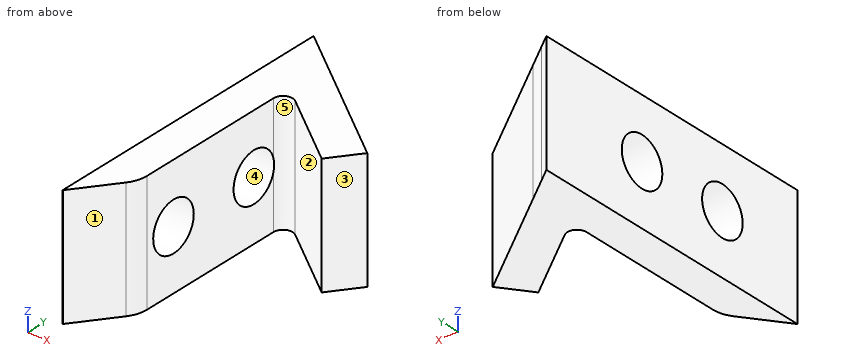
from build123d import *

# Parameters (mm, degrees)
BOSS_EXTRUDE1_DEPTH = 10
FILLET1_R           = 0.8
FILLET2_R           = 2.5
SKETCH6_R           = 2.02
CUT_EXTRUDE1_DEPTH  = 4


with BuildPart() as part:
    # Sketch2 → Boss-Extrude1 (new body)
    with BuildSketch(Plane.XY):
        Polygon((0, 21.259357975), (0, 0.022383201), (0.016670773, 0.022383201), (3, 4.02798368), (3, 19.024989439), align=None)
        Polygon((0, 22.637274757), (0, 21.259357975), (3, 19.024989439), (3, 22.765631464), (1.131871138, 24.156994247), align=None)
        Polygon((3, 22.765631464), (3, 19.024989439), (10.184363913, 13.674150545), (11.976330523, 16.080154633), align=None)
        Polygon((0, 25), (0, 22.637274757), (1.131871138, 24.156994247), align=None)
    extrude(amount=BOSS_EXTRUDE1_DEPTH)

    # Fillet1
    fillet1_edges = [part.edges().sort_by_distance(p)[0] for p in [
        (3, 19.024989439, 5),
    ]]
    fillet(fillet1_edges, radius=FILLET1_R)

    # Fillet2
    fillet2_edges = [part.edges().sort_by_distance(p)[0] for p in [
        (3, 4.02798368, 5),
    ]]
    fillet(fillet2_edges, radius=FILLET2_R)

    # Sketch6 → Cut-Extrude1 (cut)
    with BuildSketch(Plane.ZY):
        with Locations((5, 15.476622616)):
            Circle(SKETCH6_R)
        with Locations((5, 7.476622616)):
            Circle(SKETCH6_R)
    extrude(amount=-CUT_EXTRUDE1_DEPTH, mode=Mode.SUBTRACT)


solid = part.part
Design review of the part built by this model. Coordinates are the model's own, in mm. Face numbers are marked on the shaded views. A direction names the side the tool comes from. Round coordinates to 2 decimals unless told otherwise and drop trailing zeros. Write each loop counter-clockwise with the first axis right and the second up, starting at its lowest first coordinate (ties: lowest second). Pieces come first, ordered by that corner, then holes. Notation, with made-up numbers: (76, 77) -> (101, 77) arc R30 ccw to (101, 99) -> close; hole circle Ø9 at (43.25, -20). An arc over 180 degrees is marked (long way). One line per item, written item: value. Start each with the question number.
Q1. Insertion check: P1, Ø4.5, axis at y = 15.48, z = 5, coming from the +X side; P2, Ø2, axis at x = 3, z = 8.5, coming from the -Y side; P3, Ø6, axis at y = 4.5, z = 3.5, coming from the +X side. Each pin has a flat end and moves straight along its axis. Give the tip position at first contact, or say it passes through.
Q2. To check wall thickness, follow probe 1 along Y at (x, z) = (1.4, 5); probe 2 along Y at (x, z) = (2.25, 5); probe 3 along X at (y, z) = (9.5, 8). State the ranges of each line that lie inside material, in increasing order.
Q3. The part is to be moulded in two halves that separate along X. For the marked faces 3, 4 and 5, say which applies: pulls with the +X half, pulls with the -X half, needs draft (parallel to the pull), parting line crosses it, or undercut.
Q4. Add section B-B (y = 14.5). Give the boundary of the cut face in (x, z), then the cut area to 3 significant figures.
Q5. Add section D-D (z = 9.25). Give the boundary of the cut face in (x, y) (3 decimals).
Q6. Tool access review of the marked faces 1 and 2: name each direction out of +Z, -Z, +X, -X, +Y, -Y from which nothing blocks a thin tool from reaching the whole face with its end or side.
Q7. Add section C-C (y = 6). Give the boundary of the cut face in (x, z).
Q8. Add section A-A (z = 5). Give the boundary of the cut face in (x, y) (3 decimals), then the cut area to 3 significant figures.
Response:
1. P1: stops at x = 11.98
1. P2: stops at y = 2.69
1. P3: stops at x = 3
2. probe 1: y = 1.88 to 5.46, 9.5 to 13.46, 17.5 to 23.96
2. probe 2: y = 3.02 to 5.46, 9.5 to 13.46, 17.5 to 23.32
2. probe 3: x = 0 to 3
3. face 3: pulls with the +X half
3. face 4: needs draft
3. face 5: undercut
4. outline: (0, 0) -> (3, 0) -> (3, 3.23) -> (0, 3.23) -> close; (0, 6.77) -> (3, 6.77) -> (3, 10) -> (0, 10) -> close; (9.08, 0) -> (10.8, 0) -> (10.8, 10) -> (9.08, 10) -> close
4. area: 36.6 mm^2
5. outline: (0, 0.022) -> (0.017, 0.022) -> (2.505, 3.363) arc R2.5 ccw to (3, 4.857) -> (3, 17.432) arc R0.8 cw to (4.278, 18.073) -> (10.184, 13.674) -> (11.976, 16.08) -> (0, 25) -> close
6. face 1: +Z, -Z, +X, -Y
6. face 2: +Z, -Z, -Y
7. outline: (0, 0) -> (3, 0) -> (3, 3.62) -> (0, 3.62) -> close; (0, 6.38) -> (3, 6.38) -> (3, 10) -> (0, 10) -> close
8. outline: (0, 0.022) -> (0.017, 0.022) -> (2.505, 3.363) arc R2.5 ccw to (3, 4.857) -> (3, 5.457) -> (0, 5.457) -> close; (0, 9.497) -> (3, 9.497) -> (3, 13.457) -> (0, 13.457) -> close; (0, 17.497) -> (3.003, 17.497) arc R0.8 cw to (4.278, 18.073) -> (10.184, 13.674) -> (11.976, 16.08) -> (0, 25) -> close
8. area: 72.1 mm^2
